Design review of the part built by this model. Coordinates are the model's own, in mm. Coordinates: 2 decimals unless noted, no trailing zeros. Loops run counter-clockwise (first coordinate to the right, second up) from the corner with the lowest first, then second, coordinate; pieces in that order, holes last. Notation, with made-up numbers: (89.25, 80) - (109.25, 80) arc R25 ccw to (109.25, 109) - close; hole circle Ø6 at (74.25, 48). An arc over 180 degrees is marked (long way). Answer in a Markdown table with one row per item. Add a question column.
(1) We need section B-B, the plane x = 0. Write out the cut boundary in (y, z), plus the area to 3 significant figures.
(2) We need section A-A, the plane z = 0. Write out the cut boundary in (x, y), plus the area to 3 significant figures.
(3) The part is to be moulded in two halves that separate along Z. For faces 1 (the face through (-47, -2.5, -3)), 2 (the face through (4.347, -0.035, 10.485)), say which applies: released by +Z, released by -Z, zero draft, split by the parting line, or undercut.
(4) To check wall thickness, follow L1, parallel to Z at x = 0, y = 1.25; L2, parallel to X at y = 0, z = 0. State the ranges of each line that lie inside material, in increasing order. Write a range as [from, to].
Autodesk Inventor part; units mm, degrees
ref_plane "YZ Plane" through (0, 0, 0) normal (1, 0, 0) x (0, 1, 0)
ref_plane "XZ Plane" through (0, 0, 0) normal (0, 1, 0) x (-1, 0, 0)
ref_plane "XY Plane" through (0, 0, 0) normal (0, 0, 1) x (1, 0, 0)
sketch "Sketch1" plane through (0, 0, 0) normal (0, 1, 0) x (-1, 0, 0)
  line L0 (225, 317.9348) -> (-225, 317.9348)
  line L1 (-225, 317.9348) -> (-225, -332.0652)
  line L2 (-225, -332.0652) -> (225, -332.0652)
  line L3 (225, -332.0652) -> (225, 317.9348)
  point P0 (0, 0)
  dimension "d11" = 450
  dimension "d12" = 650
extrude "Extrusion1" add sketch "Sketch1" along normal mid plane 5
sketch "Sketch2" plane through (0, 2.5, 0) normal (0, 1, 0) x (1, 0, 0)
  point P0 (0, 0)
hole "Hole1" at (0, 2.5, 0) direction (0, -1, 0) diameter 22.7 end through all
properties part number "newbottom" material "PMMA Plastic"
Responses:
| question | item | result |
|---|---|---|
| 1 | outline | (-2.5, -332.07) - (2.5, -332.07) - (2.5, -11.35) - (-2.5, -11.35) - close; (-2.5, 11.35) - (2.5, 11.35) - (2.5, 317.93) - (-2.5, 317.93) - close |
| 1 | area | 3,140 mm2 |
| 2 | outline | (-225, -2.5) - (-11.35, -2.5) - (-11.35, 2.5) - (-225, 2.5) - close; (11.35, -2.5) - (225, -2.5) - (225, 2.5) - (11.35, 2.5) - close |
| 2 | area | 2,140 mm2 |
| 3 | face 1 | zero draft |
| 3 | face 2 | undercut |
| 4 | L1 | z = [-332.07, -11.35], [11.35, 317.93] |
| 4 | L2 | x = [-225, -11.35], [11.35, 225] |
